from build123d import *

# Parameters (mm, degrees)
REVOLVE1_ANGLE     = 72
CUT_EXTRUDE1_DEPTH = 10


with BuildPart() as part:
    # Sketch1 → Revolve1 (revolve)
    with BuildSketch(Plane.XY):
        with BuildLine():
            ThreePointArc((-52.157480315, 97.330708661), (-49.814334564, 102.987562911), (-44.157480315, 105.330708661))
            Line((-44.157480315, 105.330708661), (6.842519685, 105.330708661))
            ThreePointArc((6.842519685, 105.330708661), (12.499373935, 102.987562911), (14.842519685, 97.330708661))
            Line((14.842519685, 97.330708661), (14.842519685, 70.330708661))
            Line((14.842519685, 70.330708661), (10.842519685, 70.330708661))
            Line((10.842519685, 70.330708661), (10.842519685, 97.330708661))
            ThreePointArc((10.842519685, 97.330708661), (9.67094681, 100.159135786), (6.842519685, 101.330708661))
            Line((6.842519685, 101.330708661), (-44.157480315, 101.330708661))
            ThreePointArc((-44.157480315, 101.330708661), (-46.98590744, 100.159135786), (-48.157480315, 97.330708661))
            Line((-48.157480315, 97.330708661), (-48.157480315, 70.330708661))
            Line((-48.157480315, 70.330708661), (-52.157480315, 70.330708661))
            Line((-52.157480315, 70.330708661), (-52.157480315, 97.330708661))
        make_face()
    revolve(axis=Axis((14.842519685, -1144.669291339, 0), (-1, 0, 0)), revolution_arc=REVOLVE1_ANGLE)

    # Sketch2 → Cut-Extrude1 (cut)
    with BuildSketch(Plane(origin=(14.842519685, 0, 0), x_dir=(0, 0, -1), z_dir=(1, 0, 0))):
        with BuildLine():
            Line((20, 89.330708661), (32, 89.330708661))
            ThreePointArc((32, 89.330708661), (38, 83.330708661), (32, 77.330708661))
            Line((32, 77.330708661), (20, 77.330708661))
            ThreePointArc((20, 77.330708661), (14, 83.330708661), (20, 89.330708661))
        make_face()
        with BuildLine():
            Line((379.912778747, 29.563343425), (391.388435819, 26.054882969))
            ThreePointArc((391.388435819, 26.054882969), (395.372034126, 18.562824205), (387.879975362, 14.579225897))
            Line((387.879975362, 14.579225897), (376.40431829, 18.087686354))
            ThreePointArc((376.40431829, 18.087686354), (372.420719983, 25.579745118), (379.912778747, 29.563343425))
        make_face()
        with BuildLine():
            Line((706.624794334, -132.820784875), (716.573245205, -139.531099717))
            ThreePointArc((716.573245205, -139.531099717), (718.192313219, -147.860482573), (709.862930363, -149.479550587))
            Line((709.862930363, -149.479550587), (699.914479492, -142.769235746))
            ThreePointArc((699.914479492, -142.769235746), (698.295411478, -134.43985289), (706.624794334, -132.820784875))
        make_face()
        with BuildLine():
            Line((971.584524259, -383.630848012), (979.136368952, -392.95659955))
            ThreePointArc((979.136368952, -392.95659955), (978.249415529, -401.395397665), (969.810617414, -400.508444242))
            Line((969.810617414, -400.508444242), (962.258772721, -391.182692705))
            ThreePointArc((962.258772721, -391.182692705), (963.145726144, -382.74389459), (971.584524259, -383.630848012))
        make_face()
        with BuildLine():
            Line((1151.637008404, -700.948432155), (1156.132287525, -712.074638409))
            ThreePointArc((1156.132287525, -712.074638409), (1152.816823958, -719.885381097), (1145.00608127, -716.56991753))
            Line((1145.00608127, -716.56991753), (1140.510802149, -705.443711276))
            ThreePointArc((1140.510802149, -705.443711276), (1143.826265716, -697.632968588), (1151.637008404, -700.948432155))
        make_face()
    extrude(amount=-CUT_EXTRUDE1_DEPTH, mode=Mode.SUBTRACT)


solid = part.part
Input: part model. Units: mm. Frame: model coordinates. A direction names the side the tool comes from. Give positions to 0.01 mm unless a question says otherwise; leave off trailing zeros. Order: outer loops, then holes, each group sorted by start corner. A loop starts at its lowest first (then second) coordinate and runs counter-clockwise, first axis right, second up.
Q1. Section A-A on x = -20.5. Output: boundary loops of the cut face in (y, z).
Checked values:
outline: (-759.63, -1185.02) - (-758.4, -1188.82) arc R1250 ccw to (105.33, 0) - (101.33, 0) arc R1246 cw to start
Q2. Set-up query: faces 1 (the cylindrical face through (-50.185, -155.47, -705.485)), 2 (the cylindrical face through (-19.014, -130.231, -723.485)). Return all of +Z, -Z, +X, -X, +Y, -Y with unobstructed straight access to the full face (end or side cutting, diameter ignored); none if empty.
Checked values:
face 1: +Z, +X, -X, -Y
face 2: +Z, -Y
Q3. Contact query for flat-ended pins moving along their axis: pin 1 Ø1 at (x, z) = (6, -820) entering from -Y; pin 2 Ø8 at (x, y) = (-37, -252) entering from +Z; pin 3 Ø2 at (x, y) = (-0.5, -659.5) entering from -Z. Output: stop coordinate, or through.
Checked values:
pin 1: stops at y = -206.96
pin 2: stops at z = -865.16
pin 3: stops at z = -1152.42
Q4. Draft query along X for faces 3 (the flat face through (-16.02, -759.374, -1185.816)), 4 (the flat face through (-48.157, -145, -725)), 5 (the flat face through (-52.157, -141, -725)). Return one class per face: +X half, -X half, draft (parallel to the pull), parting line (faces both ways), or undercut.
Checked values:
face 3: draft
face 4: undercut
face 5: -X half
Q5. Ray query, probe 1 along X at (y, z) = (-375.5, -950.5); probe 2 along Z at (x, y) = (-34.5, -541.5); probe 3 along Y at (x, z) = (-9, -497). Return the intervals inside material, ascending.
Checked values:
probe 1: x = -52.16 to -48.16, 10.84 to 14.84
probe 2: z = -1094.85 to -1090.28
probe 3: y = -2.08 to 2.28
